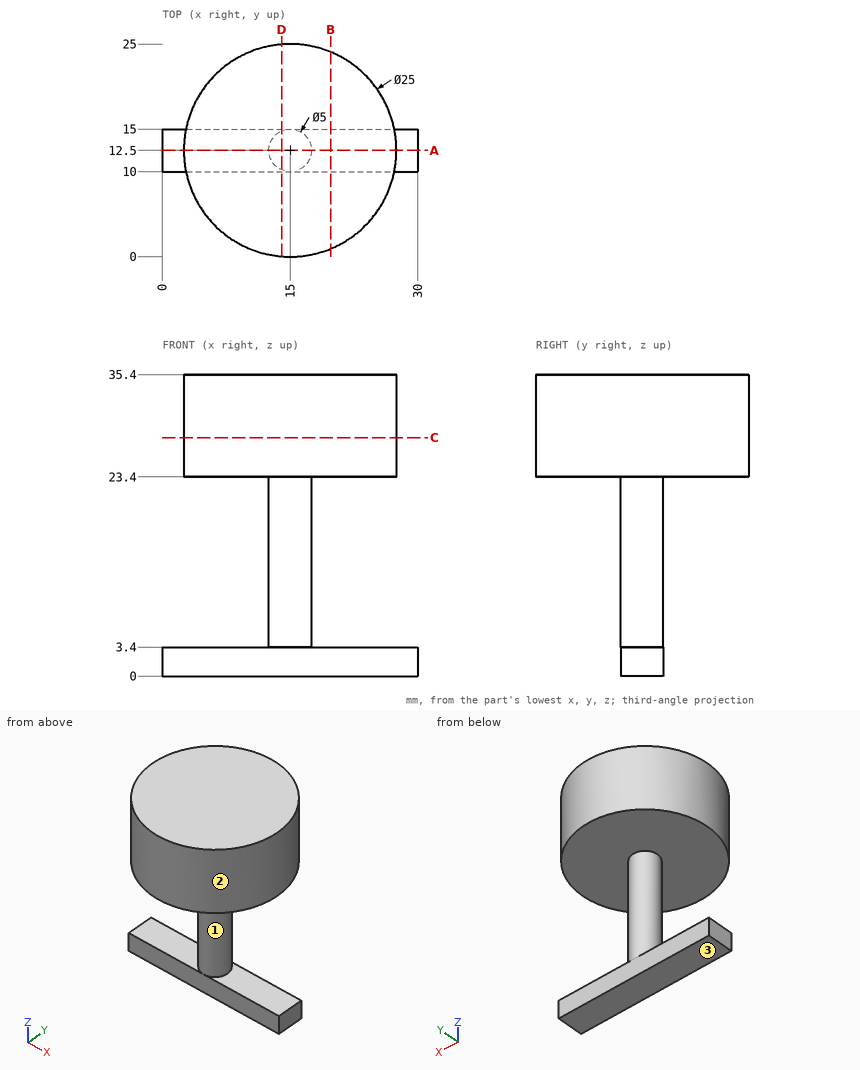
For this review, use the dimensioned drawing (mm, ordinates from the lowest corner) and the shaded views. Coordinates: 2 decimals unless noted, no trailing zeros. Loops run counter-clockwise (first coordinate to the right, second up) from the corner with the lowest first, then second, coordinate; pieces in that order, holes last. Notation, with made-up numbers: (76.25, 0) - (109.25, 0) arc R22 cw to (109.25, 28) - close; hole circle Ø9 at (22, 75). An arc over 180 degrees is marked (long way). Use CSV: the item, a comma, the result in double quotes. Start each with the question number.
1) Consider section B-B on x = 19.75. Write out the cut boundary in (y, z).
2) Consider section D-D on x = 14. Write out the cut boundary in (y, z), then the cut area to 3 significant figures.
3) For pin 1 Ø1.7 at (x, z) = (10, 1) entering from -Y; pin 2 Ø2.5 at (x, z) = (19.5, 2.5) entering from +Y; pin 3 Ø6 at (x, z) = (22.5, 30) entering from -Y; pin 4 Ø8 at (x, z) = (11, 26.5) entering from -Y, all flat-tipped, find the tip position at first contact; note any pin that passes through.
4) The part is to be moulded in two halves that separate along Z. For the marked faces 1, 2 and 3, say which applies: +Z half, -Z half, draft (parallel to the pull), parting line (faces both ways), or undercut.
5) Consider section A-A on y = 12.5. Write out the cut boundary in (x, z).
6) Wall thickness on L1, parallel to Z at x = 23, y = 12.75; L2, parallel to Z at x = 10.5, y = 17.75; L3, parallel to Z at x = 27.5, y = 14: over which ranges is each line inside the solid? List them lowest first. Write a range as from..to.
7) Consider section C-C on z = 28. Write out the cut boundary in (x, y), then the cut area to 3 significant figures.
Geometry says:
1,outline,"(0.94, 23.4) - (24.06, 23.4) - (24.06, 35.4) - (0.94, 35.4) - close; (10, 0) - (15, 0) - (15, 3.4) - (10, 3.4) - close"
2,outline,"(0.04, 23.4) - (10.21, 23.4) - (10.21, 3.4) - (10, 3.4) - (10, 0) - (15, 0) - (15, 3.4) - (14.79, 3.4) - (14.79, 23.4) - (24.96, 23.4) - (24.96, 35.4) - (0.04, 35.4) - close"
2,area,"408 mm^2"
3,pin 1,"y = 10"
3,pin 2,"y = 15"
3,pin 3,"y = 0.84"
3,pin 4,"y = 0"
4,face 1,"undercut"
4,face 2,"draft"
4,face 3,"-Z half"
5,outline,"(0, 0) - (30, 0) - (30, 3.4) - (17.5, 3.4) - (17.5, 23.4) - (27.5, 23.4) - (27.5, 35.4) - (2.5, 35.4) - (2.5, 23.4) - (12.5, 23.4) - (12.5, 3.4) - (0, 3.4) - close"
6,L1,"0..3.4, 23.4..35.4"
6,L2,"23.4..35.4"
6,L3,"0..3.4"
7,outline,"circle Ø25 at (15, 12.5)"
7,area,"491 mm^2"
